Work out the finished part from the listing and answer in its coordinate system (mm). A direction names the side the tool comes from. Give positions to 0.01 mm unless a question says otherwise; leave off trailing zeros. Order: outer loops, then holes, each group sorted by start corner. A loop starts at its lowest first (then second) coordinate and runs counter-clockwise, first axis right, second up.
```python
from build123d import *

# Parameters (mm, degrees)
SKETCH1_W           = 160.4
SKETCH1_H           = 31
SKETCH1_R           = 2.5
BOSS_EXTRUDE1_DEPTH = 2.5
BOSS_EXTRUDE2_START = -7.5
SKETCH2_R           = 4
BOSS_EXTRUDE2_DEPTH = 18
SKETCH3_W           = 14
SKETCH3_H           = 13
CUT_EXTRUDE1_DEPTH  = 18


with BuildPart() as part:
    # Sketch1 → Boss-Extrude1 (new body)
    with BuildSketch(Plane(origin=(0, 0, 0), x_dir=(1, 0, 0), z_dir=(0, 1, 0))):
        with Locations((80.2, 15.5)):
            Rectangle(SKETCH1_W, SKETCH1_H)
        with Locations((80.2, 15.5)):
            Circle(SKETCH1_R, mode=Mode.SUBTRACT)
    extrude(amount=BOSS_EXTRUDE1_DEPTH)

    # Sketch2 → Boss-Extrude2 (add)
    with BuildSketch(Plane.XY.offset(BOSS_EXTRUDE2_START)):
        with BuildLine():
            Line((20.142837701, 2.5), (50.142837701, 2.5))
            ThreePointArc((50.142837701, 2.5), (35.142837701, 17.5), (20.142837701, 2.5))
        make_face()
        with Locations((35.142837701, 9.772919339)):
            Circle(SKETCH2_R, mode=Mode.SUBTRACT)
        with BuildLine():
            Line((109.22381187, 2.5), (139.22381187, 2.5))
            ThreePointArc((139.22381187, 2.5), (124.22381187, 17.5), (109.22381187, 2.5))
        make_face()
        with Locations((124.22381187, 9.772919339)):
            Circle(SKETCH2_R, mode=Mode.SUBTRACT)
    extrude(amount=-BOSS_EXTRUDE2_DEPTH)

    # Sketch3 → Cut-Extrude1 (cut)
    with BuildSketch(Plane(origin=(0, 2.5, 0), x_dir=(1, 0, 0), z_dir=(0, 1, 0))):
        with Locations((35.142837701, 16.5)):
            Rectangle(SKETCH3_W, SKETCH3_H)
        with Locations((124.22381187, 16.5)):
            Rectangle(SKETCH3_W, SKETCH3_H)
    extrude(amount=CUT_EXTRUDE1_DEPTH, mode=Mode.SUBTRACT)


solid = part.part
```
1. Which of the six approach directions +Z, -Z, +X, -X, +Y, -Y give full straight-line access (tool end or side, diameter ignored) to faces 1 (the face through (124, 5, -25.5)), 2 (the face through (38.838, 8.241, -24.232)), 3 (the face through (127.2, 6.6, -10)), 4 (the face through (79, 0, -12)), 5 (the face through (35, 5, -7.5))?
Findings below:
face 1: -Z, +X, -X, +Y
face 2: +Z, -Z
face 3: +Y
face 4: +Z, -Z, +X, -X, -Y
face 5: +Z, +X, -X, +Y
2. Straight lines are drawn through the part: probe 1 along X at (y, z) = (10.25, -8.5); probe 2 along Z at (x, y) = (42, 4.25); probe 3 along X at (y, z) = (1.8, -15.5). For each, find the intervals that lie inside material, in ascending order.
Findings below:
probe 1: x = 22.3 to 31.17, 39.11 to 47.99, 111.38 to 120.25, 128.2 to 137.07
probe 2: z = -25.5 to -23, -10 to -7.5
probe 3: x = 0 to 77.7, 82.7 to 160.4
3. The mould has two halves that part along Z. Classify faces 6 (the face through (38.838, 8.241, -8.732)), 7 (the face through (35, 2.5, -17)), 8 (the face through (124, 5, -7.5)): pulls with the +Z half, pulls with the -Z half, needs draft (parallel to the pull), parting line crosses it, or undercut.
Findings below:
face 6: needs draft
face 7: undercut
face 8: pulls with the +Z half
4. Given P1, Ø10.5, axis at y = 12, z = -16, coming from the +X side; P2, Ø6.5, axis at y = 9, z = -17.5, coming from the -X side; P3, Ø9.5, axis at x = 60.5, z = -11, coming from the +Y side, each flat-ended and moving along its own axis, determine where each tip first touches the part or whether it passes through.
Findings below:
P1: stops at x = 138.61
P2: stops at x = 20.5
P3: stops at y = 2.5
5. The part is cut by section C-C (y = 7.5). State how many separate pieces and enclosed holes the cut face has, then the cut area to 3 significant figures.
Findings below:
separate pieces: 4
enclosed holes: 0
area: 588 mm2
6. The part is cut by section A-A (z = -15.5). Write down the section's boundary in (x, y), then the cut area to 3 significant figures.
Findings below:
outline: (0, 0) - (77.7, 0) - (77.7, 2.5) - (50.14, 2.5) arc R15 ccw to (42.14, 15.77) - (42.14, 2.5) - (28.14, 2.5) - (28.14, 15.77) arc R15 ccw to (20.14, 2.5) - (0, 2.5) - close; (82.7, 0) - (160.4, 0) - (160.4, 2.5) - (139.22, 2.5) arc R15 ccw to (131.22, 15.77) - (131.22, 2.5) - (117.22, 2.5) - (117.22, 15.77) arc R15 ccw to (109.22, 2.5) - (82.7, 2.5) - close
area: 691 mm2
7. The part is cut by section D-D (x = 125.5). Write down the section's boundary in (y, z), then the cut area to 3 significant figures.
Findings below:
outline: (0, -31) - (2.5, -31) - (2.5, -25.5) - (5.98, -25.5) - (5.98, -23) - (2.5, -23) - (2.5, -10) - (5.98, -10) - (5.98, -7.5) - (2.5, -7.5) - (2.5, 0) - (0, 0) - close; (13.56, -25.5) - (17.45, -25.5) - (17.45, -23) - (13.56, -23) - close; (13.56, -10) - (17.45, -10) - (17.45, -7.5) - (13.56, -7.5) - close
area: 114 mm2
8. The part is cut by section B-B (x = 80.2). Write down the section's boundary in (y, z).
Findings below:
outline: (0, -31) - (2.5, -31) - (2.5, -18) - (0, -18) - close; (0, -13) - (2.5, -13) - (2.5, 0) - (0, 0) - close
